Design review of the part shown in the three views and the two pictorial views. Dimensions are in mm from the part's minimum x, y and z. Give positions to 0.01 mm unless a question says otherwise; leave off trailing zeros. Loops run counter-clockwise (first coordinate to the right, second up) from the corner with the lowest first, then second, coordinate; pieces in that order, holes last. Notation, with made-up numbers: (28.25, 88) - (43.25, 88) arc R15 ccw to (43.25, 92) - close; hole circle Ø10 at (83, 68.5). An arc over 180 degrees is marked (long way). Answer in a Markdown table with one row per item.
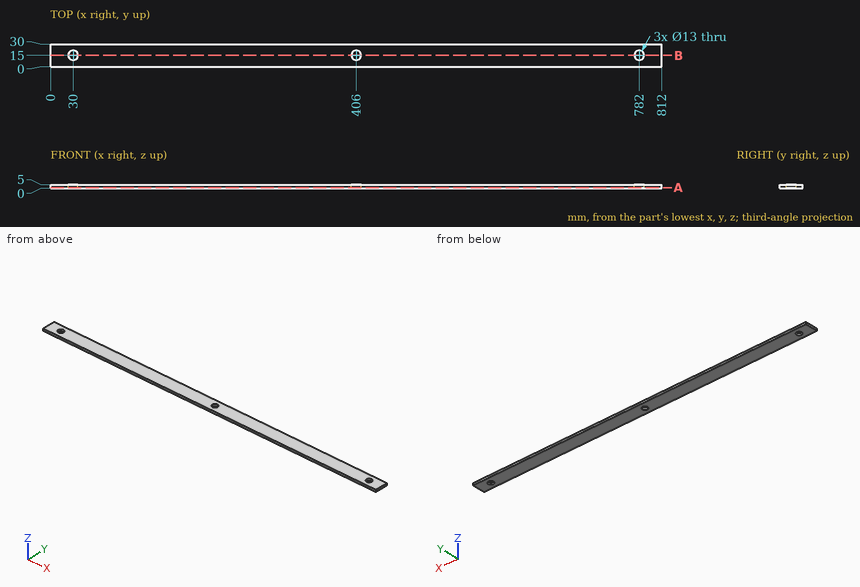
1. Clearance check with a flat-ended pin moving along its axis: pin 1 (3 mm diameter, centred on x = 170, y = 15.5, fed in from -Z). State where the tip first meets the part, or that it passes through.
Values:
| item | result |
|---|---|
| pin 1 | stops at z = 0 |
2. We need section B-B, the plane y = 15. Give the boundary of the cut face in (x, z).
Values:
| item | result |
|---|---|
| outline | (0, 0) - (23.5, 0) - (23.5, 5) - (0, 5) - close; (36.5, 0) - (399.5, 0) - (399.5, 5) - (36.5, 5) - close; (412.5, 0) - (775.5, 0) - (775.5, 5) - (412.5, 5) - close; (788.5, 0) - (812, 0) - (812, 5) - (788.5, 5) - close |
3. We need section A-A, the plane z = 0.85. Give the boundary of the cut face in (x, y), and give its area (3 significant figures).
Values:
| item | result |
|---|---|
| outline | (0, 0) - (812, 0) - (812, 30) - (0, 30) - close; hole circle Ø13 at (30, 15); hole circle Ø13 at (406, 15); hole circle Ø13 at (782, 15) |
| area | 24,000 mm^2 |
4. Wall thickness on line 1 (Y direction, x = 782, z = 3.2); line 2 (X direction, y = 9, z = 1.6); line 3 (X direction, y = 19.5, z = 4): over which ranges is each line inside the solid? List them lowest first. Write a range as [from, to].
Values:
| item | result |
|---|---|
| line 1 | y = [0, 8.5], [21.5, 30] |
| line 2 | x = [0, 27.5], [32.5, 403.5], [408.5, 779.5], [784.5, 812] |
| line 3 | x = [0, 25.31], [34.69, 401.31], [410.69, 777.31], [786.69, 812] |
